The listing builds one solid part. Answer for the finished solid, in the listing's coordinates (mm). A direction names the side the tool comes from. Round coordinates to 2 decimals unless told otherwise and drop trailing zeros. Loops run counter-clockwise (first coordinate to the right, second up) from the corner with the lowest first, then second, coordinate; pieces in that order, holes last. Notation, with made-up numbers: M -27,-30 L 8,-30 A12 ccw 8,-11 Z; hole C 31.25,69.25 d9. An arc over 180 degrees is marked long. Answer as a JSON object with one key per item and string values.
```python
from build123d import *

# Parameters (mm, degrees)
F0_W     = 127
F0_H     = 76.2
F1_DEPTH = 15.24
F3_DEPTH = 15.241
F4_T     = -3.81
F5_R     = 1.778
F6_DEPTH = 15.241


with BuildPart() as f1:
    # F0 (on Top) → F1 (new body)
    with BuildSketch(Plane.XY):
        Rectangle(F0_W, F0_H)
    extrude(amount=F1_DEPTH)

    # F2 (on Top) → F3 (cut, through all)
    with BuildSketch(Plane.XY):
        with BuildLine():
            ThreePointArc((-47.371, 28.575), (-50.8, 32.004), (-54.229, 28.575))
            Line((-54.229, 28.575), (-54.229, -28.575))
            ThreePointArc((-54.229, -28.575), (-50.8, -32.004), (-47.371, -28.575))
            Line((-47.371, -28.575), (-47.371, 28.575))
        make_face()
        with BuildLine():
            ThreePointArc((54.229, 28.575), (50.8, 32.004), (47.371, 28.575))
            Line((47.371, 28.575), (47.371, -28.575))
            ThreePointArc((47.371, -28.575), (50.8, -32.004), (54.229, -28.575))
            Line((54.229, -28.575), (54.229, 28.575))
        make_face()
    extrude(amount=F3_DEPTH, mode=Mode.SUBTRACT)

    # F4
    f4_openings = [f1.faces().sort_by_distance(p)[0] for p in [
        (0, 0, 0),
    ]]
    offset(amount=F4_T, openings=f4_openings)

    # F5 (on Top) → F6 (cut, through all)
    with BuildSketch(Plane.XY):
        with Locations((-24.765, 24.765)):
            Circle(F5_R)
        with Locations((24.765, 24.765)):
            Circle(F5_R)
        with Locations((-24.765, -24.765)):
            Circle(F5_R)
        with Locations((24.765, -24.765)):
            Circle(F5_R)
    extrude(amount=F6_DEPTH, mode=Mode.SUBTRACT)


solid = f1.part
```
Item 1: The part is cut by section B-B (y = -15.5). Give the vertices of the cut face in (x, z).
Values follow:
{"outline": "M -63.5,0 L -59.69,0 L -59.69,11.43 L -58.04,11.43 L -58.04,0 L -54.23,0 L -54.23,15.24 L -63.5,15.24 Z; M -47.37,0 L -43.56,0 L -43.56,11.43 L 43.56,11.43 L 43.56,0 L 47.37,0 L 47.37,15.24 L -47.37,15.24 Z; M 54.23,0 L 58.04,0 L 58.04,11.43 L 59.69,11.43 L 59.69,0 L 63.5,0 L 63.5,15.24 L 54.23,15.24 Z"}
Item 2: The part is cut by section D-D (x = 52). Give the vertices of the cut face in (y, z), then the cut area to 3 significant figures.
Values follow:
{"outline": "M -38.1,0 L -31.79,0 L -31.79,15.24 L -38.1,15.24 Z; M 31.79,0 L 38.1,0 L 38.1,15.24 L 31.79,15.24 Z", "area": "192 mm^2"}
Item 3: The part is cut by section A-A (x = -50.8). Give the vertices of the cut face in (y, z).
Values follow:
{"outline": "M -38.1,0 L -32,0 L -32,15.24 L -38.1,15.24 Z; M 32,0 L 38.1,0 L 38.1,15.24 L 32,15.24 Z"}
Item 4: The part is cut by section C-C (x = 38). Give the vertices of the cut face in (y, z), then the cut area to 3 significant figures.
Values follow:
{"outline": "M -38.1,0 L -34.29,0 L -34.29,11.43 L 34.29,11.43 L 34.29,0 L 38.1,0 L 38.1,15.24 L -38.1,15.24 Z", "area": "377 mm^2"}
Item 5: Which of the six approach directions +Z, -Z, +X, -X, +Y, -Y give full straight-line access (tool end or side, diameter ignored) to faces 1 (the face through (-59.69, 0, 6)), 2 (the face through (-47.371, 0, 8))?
Values follow:
{"face 1": "-Z", "face 2": "+Z, -Z"}
Item 6: Straight lines are drawn through the part: line 1 (X direction, y = 13.5, z = 11.75); line 2 (X direction, y = 13, z = 9.5); line 3 (Y direction, x = -40, z = 5.5). For each, find the intervals that lie inside material, in ascending order.
Values follow:
{"line 1": "-63.5 to -54.23, -47.37 to 47.37, 54.23 to 63.5", "line 2": "-63.5 to -59.69, -58.04 to -54.23, -47.37 to -43.56, 43.56 to 47.37, 54.23 to 58.04, 59.69 to 63.5", "line 3": "-38.1 to -34.29, 34.29 to 38.1"}
Item 7: A flat-ended cylindrical pin translates along its axis: P1, Ø5, axis at x = 2, y = 2, coming from the -Z side. Find the tip coordinate at first contact, or state that the pin passes through.
Values follow:
{"P1": "z = 11.43"}
Item 8: Determine the mould class of faces 3 (the face through (51, -32, 8)), 4 (the face through (-51, -32, 8)), 5 (the face through (0, 37, 0)) for opening direction X: released by +X, released by -X, zero draft, split by the parting line, or undercut.
Values follow:
{"face 3": "undercut", "face 4": "undercut", "face 5": "zero draft"}
